Input: part model. Units: mm. Frame: model coordinates. A direction names the side the tool comes from. Coordinates: 2 decimals unless noted, no trailing zeros. Loops run counter-clockwise (first coordinate to the right, second up) from the corner with the lowest first, then second, coordinate; pieces in that order, holes last. Notation, with made-up numbers: (-12.5, 10) - (38.5, 10) arc R32 ccw to (38.5, 43) - close; hole circle Ø7 at (50.5, 6.25). An arc over 180 degrees is marked (long way). Use one line per item in the form item = value.
from build123d import *

# Parameters (mm, degrees)
F0_R     = 12.7
F1_DEPTH = 12.7
F2_W     = 12.7
F2_H     = 101.6
F3_DEPTH = 25.4
F2_W_2   = 25.4
F4_DEPTH = 76.2
F5_R     = 12.7
F6_DEPTH = 25.4
F7_W     = 24.888192
F7_H     = 88.9
F8_DEPTH = 25.4


with BuildPart() as f1:
    # F0 (on Top) → F1 (new body)
    with BuildSketch(Plane.XY):
        Polygon((-38.1, -50.8), (38.1, -50.8), (38.1, 50.8), (-38.1, 50.8), (-63.5, 50.8), (-63.5, -25.4), (-38.1, -25.4), align=None)
        with Locations((-38.1, 12.7)):
            Circle(F0_R, mode=Mode.SUBTRACT)
    extrude(amount=F1_DEPTH)

    # F2 (on face) → F3 (cut)
    with BuildSketch(Plane.XY.offset(12.7)):
        with Locations((31.75, 0)):
            Rectangle(F2_W, F2_H)
    extrude(amount=-F3_DEPTH, mode=Mode.SUBTRACT)

    # F2 (on face) → F4 (join)
    with BuildSketch(Plane.XY.offset(12.7)):
        with Locations((12.7, 0)):
            Rectangle(F2_W_2, F2_H)
    extrude(amount=F4_DEPTH)

    # F5 (on face) → F6 (cut)
    with BuildSketch(Plane.YZ.offset(25.4)):
        with Locations((-12.7, 63.5)):
            Circle(F5_R)
    extrude(amount=-F6_DEPTH, mode=Mode.SUBTRACT)

    # F7 (on face) → F8 (join)
    with BuildSketch(Plane.YZ.offset(25.4)):
        with Locations((38.355904, 44.45)):
            Rectangle(F7_W, F7_H)
    extrude(amount=F8_DEPTH)


solid = f1.part
Q1. Ray query, line 1 along X through (y, z) = (12, 4); line 2 along Z through (x, y) = (13, -12); line 3 along Y through (x, z) = (17, 63). Return the intervals inside material, ascending. Write a range as [from, to].
Check values:
line_1 = [-63.5, -50.78], [-25.42, 25.4]
line_2 = [0, 50.82], [76.18, 88.9]
line_3 = [-50.8, -25.39], [-0.01, 50.8]
Q2. Pull-direction query (Y, two-part tool) for faces 1 (the cylindrical face through (12.878, -0.586, 67.315)), 2 (the flat face through (18, 50.8, 44)), 3 (the flat face through (-63.5, 13, 6)); classes: pulls with the +Y half, pulls with the -Y half, needs draft (parallel to the pull), parting line crosses it, or undercut.
Check values:
face_1 = undercut
face_2 = pulls with the +Y half
face_3 = needs draft
Q3. Cut plane B-B, the plane y = 12.7. Return loops of the section in (x, z).
Check values:
outline = (-63.5, 0) - (-50.8, 0) - (-50.8, 12.7) - (-63.5, 12.7) - close; (-25.4, 0) - (25.4, 0) - (25.4, 88.9) - (0, 88.9) - (0, 12.7) - (-25.4, 12.7) - close
Q4. Cut plane C-C, the plane y = 29. Return loops of the section in (x, z), then the cut area to 3 significant figures.
Check values:
outline = (-63.5, 0) - (50.8, 0) - (50.8, 88.9) - (0, 88.9) - (0, 12.7) - (-63.5, 12.7) - close
area = 5,320 mm²
Q5. Cut plane A-A, the plane z = 63.5. Return loops of the section in (x, y), then the cut area to 3 significant figures.
Check values:
outline = (0, -50.8) - (25.4, -50.8) - (25.4, -25.4) - (0, -25.4) - close; (0, 0) - (25.4, 0) - (25.4, 25.91) - (50.8, 25.91) - (50.8, 50.8) - (0, 50.8) - close
area = 2,570 mm²
Q6. Cut plane D-D, the plane z = 22.5. Return loops of the section in (x, y).
Check values:
outline = (0, -50.8) - (25.4, -50.8) - (25.4, 25.91) - (50.8, 25.91) - (50.8, 50.8) - (0, 50.8) - close
Q7. Set-up query: faces 4 (the flat face through (-38.1, -38, 6)), 5 (the flat face through (0, -1, 50)), 6 (the flat face through (38, 25.912, 44)). Return all of +Z, -Z, +X, -X, +Y, -Y with unobstructed straight access to the full face (end or side cutting, diameter ignored); none if empty.
Check values:
face_4 = +Z, -Z, -X, -Y
face_5 = +Z, -X, +Y, -Y
face_6 = +Z, -Z, +X, -Y
Q8. First-contact query: P1, Ø6.5, axis at y = -35, z = 4.5, coming from the -X side; P2, Ø2, axis at x = -37, y = -6, coming from the +Z side; P3, Ø10, axis at x = -49.5, z = 9.5, coming from the -Y side. Flat tips, straight axial feed; report the tip coordinate or a pass-through.
Check values:
P1 = -38.1
P2 = 12.7
P3 = -25.4
